Source: CAD feature listing. Evaluate the final solid. Frame: model axes, mm. Coordinates: 2 decimals unless noted, no trailing zeros. Answer as CSV lines item,"result".
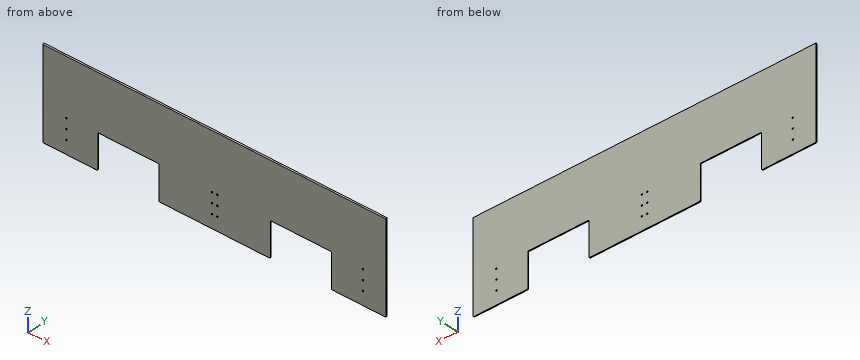
from build123d import *

# Parameters (mm, degrees)
SKETCH1_W                    = 1212.85
SKETCH1_H                    = 316.23
BOSS_EXTRUDE1_DEPTH          = 3.175
FILLET1_R                    = 3.175
SKETCH4_W                    = 215.9
SKETCH4_H                    = 120.65
CUT_EXTRUDE1_DEPTH           = 1254.402016922
FILLET2_R                    = 3.175
F_10_0_1935_DIAMETER_HOLE1_D = 4.9149


with BuildPart() as part:
    # Sketch1 → Boss-Extrude1 (new body)
    with BuildSketch(Plane(origin=(0, 0, 0), x_dir=(1, 0, 0), z_dir=(0, 1, 0))):
        with Locations((606.425, 158.115)):
            Rectangle(SKETCH1_W, SKETCH1_H)
    extrude(amount=BOSS_EXTRUDE1_DEPTH)

    # Fillet1
    fillet1_edges = [part.edges().sort_by_distance(p)[0] for p in [
        (606.425, 0, 0),
    ]]
    fillet(fillet1_edges, radius=FILLET1_R - 0.0001)  # a hair under: the kernel refuses the full size

    # Sketch4 → Cut-Extrude1 (cut, through all)
    with BuildSketch(Plane(origin=(0, 3.175, 0), x_dir=(1, 0, 0), z_dir=(0, 1, 0))):
        with Locations((301.625, 255.905)):
            Rectangle(SKETCH4_W, SKETCH4_H)
        with Locations((911.225, 255.905)):
            Rectangle(SKETCH4_W, SKETCH4_H)
    extrude(amount=-CUT_EXTRUDE1_DEPTH, mode=Mode.SUBTRACT)

    # Fillet2
    fillet2_edges = [part.edges().sort_by_distance(p)[0] for p in [
        (193.675, 1.5875, -195.58),
        (193.675, 1.5875, -316.23),
        (409.575, 1.5875, -316.23),
        (409.575, 1.5875, -195.58),
        (803.275, 1.5875, -316.23),
        (1019.175, 1.5875, -316.23),
        (1019.175, 1.5875, -195.58),
        (803.275, 1.5875, -195.58),
        (0, 1.5875, -316.23),
        (1212.85, 1.5875, -316.23),
    ]]
    fillet(fillet2_edges, radius=FILLET2_R)

    # #10 (0.1935) Diameter Hole1 (through all)
    with Locations(Plane(origin=(0, 3.175, 0), x_dir=(1, 0, 0), z_dir=(0, 1, 0))):
        with Locations((82.55, 200.1012), (82.55, 235.0262), (82.55, 269.9512), (596.9, 200.1012), (596.9, 235.0262), (596.9, 269.9512), (615.95, 269.9512), (615.95, 235.0262), (615.95, 200.1012), (1130.3, 269.9512), (1130.3, 235.0262), (1130.3, 200.1012)):
            Hole(F_10_0_1935_DIAMETER_HOLE1_D / 2)


solid = part.part
(1) Pin query (flat end, axial travel): pin 1 Ø1.5 at (x, y) = (1032, 1) entering from +Z; pin 2 Ø3 at (x, z) = (1130.3, -235.03) entering from -Y. Return the tip coordinate at first contact, or that it passes through.
Computed values:
pin 1,"z = -0.34"
pin 2,"through"
(2) Cut plane A-A (y = 0.5). State how many separate pieces and enclosed holes the cut face has, then the cut area to 3 significant figures.
Computed values:
separate pieces,"1"
enclosed holes,"12"
area,"329,000 mm^2"
(3) Material intervals for L1, parallel to X at y = 1.3, z = -256 (3 decimals); L2, parallel to Z at x = 1130, y = 2.85; L3, parallel to Z at x = 82.55, y = 2.55, sorted ascending. Write a range as [from, to].
Computed values:
L1,"[0, 193.675], [409.575, 803.275], [1019.175, 1212.85]"
L2,"[-316.23, -272.39], [-267.51, -237.47], [-232.59, -202.54], [-197.66, -0.02]"
L3,"[-316.23, -272.41], [-267.49, -237.48], [-232.57, -202.56], [-197.64, -0.06]"
